```python
from build123d import *

# Parameters (mm, degrees)
SKETCH2_W           = 70
SKETCH2_H           = 30
BOSS_EXTRUDE1_DEPTH = 4
SKETCH4_W           = 40
SKETCH4_H           = 25
BOSS_EXTRUDE7_DEPTH = 75
SKETCH6_W           = 22.4
SKETCH6_H           = 15
CUT_EXTRUDE13_DEPTH = 76.5
SKETCH8_W           = 22.8
SKETCH8_H           = 65
CUT_EXTRUDE14_DEPTH = 17
SKETCH9_R           = 1.25
CUT_EXTRUDE15_DEPTH = 28.5
SKETCH10_R          = 2.9
CUT_EXTRUDE18_DEPTH = 10
SKETCH11_W          = 5
SKETCH11_H          = 2.8
CUT_EXTRUDE17_DEPTH = 10
SKETCH12_R          = 1.25
CUT_EXTRUDE20_DEPTH = 10


with BuildPart() as part:
    # Sketch2 → Boss-Extrude1 (new body)
    with BuildSketch(Plane.XY):
        with Locations((11.210953405, 2.8125)):
            Rectangle(SKETCH2_W, SKETCH2_H)
    extrude(amount=BOSS_EXTRUDE1_DEPTH)

    # Sketch4 → Boss-Extrude7 (add)
    with BuildSketch(Plane.XY.offset(4)):
        with Locations((11.210953405, 2.8125)):
            Rectangle(SKETCH4_W, SKETCH4_H)
    extrude(amount=BOSS_EXTRUDE7_DEPTH)

    # Sketch6 → Cut-Extrude13 (cut)
    with BuildSketch(Plane(origin=(0, 0, 0), x_dir=(-1, 0, 0), z_dir=(0, 0, -1))):
        with Locations((-11.210953405, 2.8125)):
            Rectangle(SKETCH6_W, SKETCH6_H)
    extrude(amount=-CUT_EXTRUDE13_DEPTH, mode=Mode.SUBTRACT)

    # Sketch8 → Cut-Extrude14 (cut)
    with BuildSketch(Plane(origin=(0, 15.3125, 0), x_dir=(1, 0, 0), z_dir=(0, 1, 0))):
        with Locations((11.210953405, -41.5)):
            Rectangle(SKETCH8_W, SKETCH8_H)
    extrude(amount=-CUT_EXTRUDE14_DEPTH, mode=Mode.SUBTRACT)

    # Sketch9 → Cut-Extrude15 (cut, through all)
    with BuildSketch(Plane(origin=(0, 15.3125, 0), x_dir=(1, 0, 0), z_dir=(0, 1, 0))):
        with Locations((-6.289046595, -9)):
            Circle(SKETCH9_R)
        with Locations((28.710953405, -9)):
            Circle(SKETCH9_R)
        with Locations((-6.289046595, -74)):
            Circle(SKETCH9_R)
        with Locations((28.710953405, -74)):
            Circle(SKETCH9_R)
    extrude(amount=-CUT_EXTRUDE15_DEPTH, mode=Mode.SUBTRACT)

    # Sketch10 → Cut-Extrude18 (cut)
    with BuildSketch(Plane.XZ.offset(9.6875)):
        with Locations((11.210953405, 59)):
            Circle(SKETCH10_R)
    extrude(amount=-CUT_EXTRUDE18_DEPTH, mode=Mode.SUBTRACT)

    # Sketch11 → Cut-Extrude17 (cut)
    with BuildSketch(Plane.XY.offset(79)):
        with Locations((11.210953405, 5.2125)):
            Rectangle(SKETCH11_W, SKETCH11_H)
    extrude(amount=-CUT_EXTRUDE17_DEPTH, mode=Mode.SUBTRACT)

    # Sketch12 → Cut-Extrude20 (cut)
    with BuildSketch(Plane(origin=(0, 0, 0), x_dir=(-1, 0, 0), z_dir=(0, 0, -1))):
        with Locations((-41.210953405, 15.3125)):
            Circle(SKETCH12_R)
        with Locations((18.789046595, 15.3125)):
            Circle(SKETCH12_R)
        with Locations((18.789046595, -9.6875)):
            Circle(SKETCH12_R)
        with Locations((-41.210953405, -9.6875)):
            Circle(SKETCH12_R)
    extrude(amount=-CUT_EXTRUDE20_DEPTH, mode=Mode.SUBTRACT)


solid = part.part
```
Source: CAD feature listing. Evaluate the final solid. Frame: model axes, mm. A direction names the side the tool comes from. Coordinates: 2 decimals unless noted, no trailing zeros. Write each loop counter-clockwise with the first axis right and the second up, starting at its lowest first coordinate (ties: lowest second). Pieces come first, ordered by that corner, then holes. Notation, with made-up numbers: M -27,-26 L -2,-26 A36 cw -2,12 Z; hole C 18,87 d9. An arc over 180 degrees is marked long. Answer as a JSON object with one key per item and string values.
1. Contact query for flat-ended pins moving along their axis: P1, Ø6, axis at x = 33, z = 15.5, coming from the +Y side; P2, Ø2, axis at x = 10.5, z = 78.5, coming from the -Y side; P3, Ø4.5, axis at y = 1, z = 21, coming from the -X side; P4, Ø2, axis at x = 41.21, y = 15.31, coming from the -Z side. Output: stop coordinate, or through.
Evaluation:
{"P1": "y = 15.31", "P2": "y = -9.69", "P3": "x = -8.79", "P4": "through"}
2. Ray query, L1, parallel to Z at x = 28.5, y = 13.5; L2, parallel to Y at x = 4, z = 6; L3, parallel to Z at x = 10, y = 10.5. Return the intervals inside material, ascending.
Evaluation:
{"L1": "0 to 7.77, 10.23 to 72.77, 75.23 to 79", "L2": "-9.69 to -4.69, 10.31 to 15.31", "L3": "0 to 9, 74 to 79"}
3. Access query for faces 1 (the flat face through (22.411, -3, 32)), 2 (the flat face through (24, 15.312, 41)), 3 (the flat face through (8.711, 5, 78)). Directions: +Z, -Z, +X, -X, +Y, -Y. A direction counts if a zero-diameter tool reaches every point of the face in a straight line with its end or side. Return the directions, or none.
Evaluation:
{"face 1": "-Z", "face 2": "+Z, +X, -X, +Y", "face 3": "+Z, -Z"}
4. Cut plane B-B on x = 3. Output: boundary loops of the cut face in (y, z).
Evaluation:
{"outline": "M -12.19,0 L -4.69,0 L -4.69,76.5 L 10.31,76.5 L 10.31,74 L 15.31,74 L 15.31,79 L -9.69,79 L -9.69,4 L -12.19,4 Z; M 10.31,0 L 17.81,0 L 17.81,4 L 15.31,4 L 15.31,9 L 10.31,9 Z"}
5. Cut plane C-C on y = 1. Output: boundary loops of the cut face in (x, z), plus the area to 3 significant figures.
Evaluation:
{"outline": "M -23.79,0 L 0.01,0 L 0.01,9 L -0.19,9 L -0.19,74 L 0.01,74 L 0.01,76.5 L 22.41,76.5 L 22.41,74 L 22.61,74 L 22.61,9 L 22.41,9 L 22.41,0 L 46.21,0 L 46.21,4 L 31.21,4 L 31.21,79 L -8.79,79 L -8.79,4 L -23.79,4 Z; hole C -6.29,9 d2.5; hole C -6.29,74 d2.5; hole C 28.71,9 d2.5; hole C 28.71,74 d2.5", "area": "1,520 mm^2"}
6. Draft query along Y for faces 4 (the flat face through (11, -12.188, 2)), 5 (the flat face through (-8.789, 3, 41)), 6 (the flat face through (11, 3, 76.5)), 7 (the flat face through (11, 6.613, 78)). Return one class per face: released by +Y, released by -Y, zero draft, split by the parting line, or undercut.
Evaluation:
{"face 4": "released by -Y", "face 5": "zero draft", "face 6": "undercut", "face 7": "undercut"}
7. Cut plane A-A on z = 59. Output: boundary loops of the cut face in (x, y), plus the area to 3 significant figures.
Evaluation:
{"outline": "M -8.79,-9.69 L 8.31,-9.69 L 8.31,-4.69 L 0.01,-4.69 L 0.01,-1.69 L -0.19,-1.69 L -0.19,15.31 L -8.79,15.31 Z; M 14.11,-9.69 L 31.21,-9.69 L 31.21,15.31 L 22.61,15.31 L 22.61,-1.69 L 22.41,-1.69 L 22.41,-4.69 L 14.11,-4.69 Z", "area": "516 mm^2"}
8. Cut plane D-D on z = 69.5. Output: boundary loops of the cut face in (x, y).
Evaluation:
{"outline": "M -8.79,-9.69 L 31.21,-9.69 L 31.21,15.31 L 22.61,15.31 L 22.61,-1.69 L 22.41,-1.69 L 22.41,-4.69 L 0.01,-4.69 L 0.01,-1.69 L -0.19,-1.69 L -0.19,15.31 L -8.79,15.31 Z"}
